```python
from build123d import *

# Parameters (mm, degrees)
BOSS_EXTRUDE1_DEPTH = 2
FILLET1_R           = 2


with BuildPart() as part:
    # Sketch2 → Boss-Extrude1 (new body)
    with BuildSketch(Plane(origin=(0, 0, 0), x_dir=(1, 0, 0), z_dir=(0, 1, 0))):
        Polygon((-50, 45), (50, 45), (50, 8), (30, 8), (30, -8), (50, -8), (50, -45), (-50, -45), (-50, -8), (-30, -8), (-30, 8), (-50, 8), align=None)
    extrude(amount=BOSS_EXTRUDE1_DEPTH)

    # Fillet1
    fillet1_edges = [part.edges().sort_by_distance(p)[0] for p in [
        (-50, 1, -45),
        (50, 1, -45),
        (50, 1, -8),
        (30, 1, -8),
        (30, 1, 8),
        (50, 1, 8),
        (50, 1, 45),
        (-50, 1, 45),
        (-50, 1, 8),
        (-30, 1, 8),
        (-30, 1, -8),
        (-50, 1, -8),
    ]]
    fillet(fillet1_edges, radius=FILLET1_R)


solid = part.part
```
Check sheet for the modelled part. Datum: model origin and axes. Units: mm. Round coordinates to 2 decimals unless told otherwise and drop trailing zeros. Order: outer loops, then holes, each group sorted by start corner. A loop starts at its lowest first (then second) coordinate and runs counter-clockwise, first axis right, second up. Notation, with made-up numbers: (50.5, -9.5) - (67.5, -9.5) arc R16 ccw to (67.5, 0.5) - close; hole circle Ø8 at (57.25, 49). An arc over 180 degrees is marked (long way). Answer as CSV lines item,"result". Start each with the question number.
1) Depth check by flat-ended pin: pin 1 (1 mm diameter, centred on y = 0.5, z = 1, fed in from +X). Enter the tip coordinate at first touch or a pass-through.
2) Scan lines: probe 1 along Z at (x, y) = (46, 0.65); probe 2 along X at (y, z) = (0.7, 0.5). Record each from-to range of solid material in increasing order.
3) Section check A-A (x = 36). Record the cut outline in (y, z), then the cut area to 3 significant figures.
4) Section check B-B (y = 0.65). Record the cut outline in (x, z), then the cut area to 3 significant figures.
Determined:
1,pin 1,"x = 30"
2,probe 1,"-45 to -8, 8 to 45"
2,probe 2,"-30 to 30"
3,outline,"(0, -45) - (2, -45) - (2, -8) - (0, -8) - close; (0, 8) - (2, 8) - (2, 45) - (0, 45) - close"
3,area,"148 mm^2"
4,outline,"(-50, -43) arc R2 ccw to (-48, -45) - (48, -45) arc R2 ccw to (50, -43) - (50, -10) arc R2 ccw to (48, -8) - (32, -8) arc R2 cw to (30, -6) - (30, 6) arc R2 cw to (32, 8) - (48, 8) arc R2 ccw to (50, 10) - (50, 43) arc R2 ccw to (48, 45) - (-48, 45) arc R2 ccw to (-50, 43) - (-50, 10) arc R2 ccw to (-48, 8) - (-32, 8) arc R2 cw to (-30, 6) - (-30, -6) arc R2 cw to (-32, -8) - (-48, -8) arc R2 ccw to (-50, -10) - close"
4,area,"8,360 mm^2"
